Check sheet for the modelled part. Datum: model origin and axes. Units: mm. A direction names the side the tool comes from. Coordinates: 2 decimals unless noted, no trailing zeros. Order: outer loops, then holes, each group sorted by start corner. A loop starts at its lowest first (then second) coordinate and runs counter-clockwise, first axis right, second up.
1. Thickness scan on line 1 (X direction, y = 40, z = -17); line 2 (X direction, y = 68, z = 24); line 3 (Z direction, x = 15, y = 27). Record the ranges inside material, lowest first.
2. Cross-section at C-C (y = 46). Enter the section's corners in (x, z), then the cut area to 3 significant figures.
3. Cross-section at B-B (x = -26). Enter the section's corners in (y, z), then the cut area to 3 significant figures.
4. Cross-section at D-D (z = -24.5). Enter the section's corners in (x, y).
5. Set-up check for faces 5 (the flat face through (-24.669, 32, -5)), 6 (the flat face through (10, 8, 31.058)), 7 (the flat face through (-10, 23, -9.468)): record each of +Z, -Z, +X, -X, +Y, -Y from which the full face is reachable in a straight line by a thin tool's end or side.
6. Gauge pin test, flat ends, axial feed: pin 1 Ø8 at (y, z) = (22.5, -18) entering from -X; pin 2 Ø2 at (x, z) = (-22, 27) entering from +Y; pin 3 Ø2.5 at (x, z) = (-22.67, -36.97) entering from +Y. Record the tip position at first contact, or that the pin passes through.
7. Draft check along Y on faces 1 (the flat face through (44.331, 6, 26)), 2 (the cylindrical face through (-28.725, 52.482, -3.451)), 3 (the flat face through (39, 63, -5)), 4 (the flat face through (10, 63, -45)). Enter one of: released by +Y, released by -Y, zero draft, split by the parting line, or undercut.
8. Cross-section at A-A (x = 12). Enter the section's corners in (y, z).
Autodesk Inventor part; units mm, degrees
ref_plane "YZ Plane" through (0, 0, 0) normal (1, 0, 0) x (0, 1, 0)
ref_plane "XZ Plane" through (0, 0, 0) normal (0, 1, 0) x (-1, 0, 0)
ref_plane "XY Plane" through (0, 0, 0) normal (0, 0, 1) x (1, 0, 0)
sketch "Sketch1" plane through (0, 0, 0) normal (0, 1, 0) x (-1, 0, 0)
  line L0 (32.6686, 38.0315) -> (-52.3314, 38.0315)
  line L1 (-52.3314, 38.0315) -> (-52.3314, -46.9685)
  line L2 (-52.3314, -46.9685) -> (32.6686, -46.9685)
  line L3 (32.6686, -46.9685) -> (32.6686, 38.0315)
  point P0 (0, 0)
  dimension "d0" = 85
  dimension "d1" = 85
extrude "Extrusion1" add sketch "Sketch1" along normal blind 73
sketch "Sketch2" plane through (52.3314, 0, 38.0315) normal (1, 0, 0) x (0, 0, -1)
  point P0 (38.0315, 0)
sketch "Sketch3" plane through (52.3314, 0, 38.0315) normal (1, 0, 0) x (0, 0, -1)
  circle A0 centre (42.5, 23) radius 29.5
  line L0 (0, 73) -> (85, 73)
  line L1 (85, 0) -> (85, 73)
  point P0 (38.0315, 0)
  dimension "d4" = 59
  dimension "d5" = 50
  dimension "d6" = 42.5
extrude "Extrusion2" cut sketch "Sketch3" against normal blind 8
sketch "Sketch4" plane through (-32.6686, 0, -46.9685) normal (-1, 0, 0) x (0, 0, 1)
  arc A0 (60.973, 0) -> (24.027, 0) centre (42.5, 23) ccw
  circle A1 centre (42.5, 23) radius 29.5
  point P0 (46.9685, 0)
  point P1 (24.027, 0)
extrude "Extrusion3" cut sketch "Sketch4" against normal blind 8
sketch "Sketch5" plane through (0, 0, 0) normal (0, -1, 0) x (1, 0, 0)
  line L0 (-24.6686, 14.0044) -> (-24.6686, -22.9415)
  line L1 (-24.6686, -9.4685) -> (5.3314, -9.4685)
  line L2 (5.3314, -9.4685) -> (5.3314, 0.5315)
  line L3 (-4.6686, 0.5315) -> (-24.6686, 0.5315)
  line L4 (-24.6686, 0.5315) -> (-24.6686, -9.4685)
  line L5 (-4.6686, 0.5315) -> (-4.6686, 25.5315)
  line L6 (-4.6686, 25.5315) -> (5.3314, 25.5315)
  line L7 (5.3314, 25.5315) -> (5.3314, 0.5315)
  line L8 (-24.6686, -9.4685) -> (-24.6686, 0.5315)
  line L9 (44.3314, -9.4685) -> (14.3314, -9.4685)
  line L10 (14.3314, -9.4685) -> (14.3314, 0.5315)
  line L11 (24.1898, 0.5315) -> (44.3314, 0.5315)
  line L12 (24.1898, 0.5315) -> (24.3314, 25.5315)
  line L13 (24.3314, 25.5315) -> (14.3314, 25.5315)
  line L14 (14.3314, 25.5315) -> (14.3314, 0.5315)
  line L15 (44.3314, -9.4685) -> (44.3314, 0.5315)
  line L16 (44.3314, -22.9415) -> (44.3314, 14.0044)
  point P0 (0, 0)
  dimension "d13" = 13.473
  dimension "d35" = 10
  dimension "d36" = 9
  dimension "d37" = 10
sketch "Sketch6" plane through (-24.6686, 0, -46.9685) normal (-1, 0, 0) x (0, 0, 1)
  arc A0 (60.973, 0) -> (24.027, 0) centre (42.5, 23) ccw
  line L0 (42.5, 23) -> (131.4973, 23)
  point P0 (46.9685, 0)
extrude "Extrusion4" cut sketch "Sketch5" against normal blind 29
sketch "Sketch7" plane through (0, 0, 0) normal (0, -1, 0) x (1, 0, 0)
  line L0 (-24.6686, -22.9415) -> (44.3314, -22.9415)
  line L1 (44.3314, -22.9415) -> (44.3314, 31.0585)
  line L2 (44.3314, 31.0585) -> (-24.6686, 31.0585)
  line L3 (-24.6686, 31.0585) -> (-24.6686, -22.9415)
  point P0 (0, 0)
  dimension "d19" = 69
  dimension "d20" = 54
extrude "Extrusion5" cut sketch "Sketch7" against normal blind 17
sketch "Sketch8" plane through (0, 17, 0) normal (0, -1, 0) x (1, 0, 0)
  circle A0 centre (-15.6686, -13.9415) radius 2
  circle A1 centre (-15.6686, 11.0585) radius 2
  circle A2 centre (34.3314, 11.0585) radius 2
  circle A3 centre (34.3314, -13.9415) radius 2
  line L0 (-26.1879, -23.917) -> (41.8121, -23.917)
  line L1 (-24.6686, 31.0585) -> (44.3314, 31.0585)
  line L2 (-24.6686, 31.0585) -> (44.3314, 31.0585)
  line L3 (44.3314, 31.0585) -> (44.3314, -22.9415)
  line L4 (44.3314, -22.9415) -> (-24.6686, -22.9415)
  line L5 (-24.6686, -22.9415) -> (-24.6686, 31.0585)
  point P0 (0, 0)
  point P1 (-18.7833, -12.5016)
  dimension "d23" = 4
  dimension "d24" = 4
  dimension "d25" = 4
  dimension "d26" = 4
  dimension "d27" = 50
  dimension "d28" = 25
  dimension "d31" = 9
  dimension "d32" = 9
extrude "Extrusion6" cut sketch "Sketch8" against normal blind 5.8 contours A0 | A1 | A2 | A3
sketch "Sketch9" plane through (0, 29, 0) normal (0, -1, 0) x (1, 0, 0)
  line L0 (24.1898, 0.5315) -> (24.3314, 25.5315)
  line L1 (14.3314, 25.5315) -> (14.3314, -9.4685)
  line L2 (24.3314, 25.5315) -> (14.3314, 25.5315)
  line L3 (14.3314, 25.5315) -> (14.3314, 19.5315)
  line L4 (14.3314, 19.5315) -> (24.3314, 19.5315)
  line L5 (24.3314, 19.5315) -> (24.3314, 25.5315)
  line L6 (5.3314, -9.4685) -> (5.3314, 25.5315)
  line L7 (5.3314, 25.5315) -> (-14.6686, 25.5315)
  line L8 (-14.6686, 25.5315) -> (-14.6686, 19.5315)
  line L9 (-14.6686, 19.5315) -> (5.3314, 19.5315)
  line L10 (5.3314, 19.5315) -> (5.3314, 25.5315)
  point P0 (0, 0)
  point P1 (24.2974, 19.5315)
  dimension "d39" = 20
  dimension "d40" = 6
  dimension "d47" = 10
extrude "Extrusion7" cut sketch "Sketch9" against normal blind 61.25 contours L4 L1 L2 L0 | L9 L8 L7 L6
sketch "Sketch10" plane through (0, 73, 0) normal (0, 1, 0) x (1, 0, 0)
  line L0 (52.3314, 46.9685) -> (-32.6686, 46.9685)
  line L1 (-10.1686, 46.9685) -> (29.8314, 46.9685)
  line L2 (29.8314, 46.9685) -> (29.8314, -35.0315)
  line L3 (29.8314, -35.0315) -> (-10.1686, -35.0315)
  line L4 (-10.1686, -35.0315) -> (-10.1686, 46.9685)
  line L5 (-32.6686, 46.9685) -> (-32.6686, -38.0315)
  point P0 (0, 0)
  dimension "d43" = 40
  dimension "d44" = 82
  dimension "d51" = 22.5
sketch "Sketch11" plane through (0, 29, 0) normal (0, -1, 0) x (1, 0, 0)
  line L0 (24.2974, 19.5315) -> (14.3314, 19.5315)
  line L1 (14.3314, 19.5315) -> (34.3314, 19.5315)
  line L2 (34.3314, 19.5315) -> (34.3314, 25.5315)
  line L3 (34.3314, 25.5315) -> (14.3314, 25.5315)
  line L4 (14.3314, 25.5315) -> (14.3314, 19.5315)
  point P0 (0, 0)
  dimension "d48" = 20
extrude "Extrusion8" cut sketch "Sketch11" against normal blind 61.25
extrude "Extrusion9" cut sketch "Sketch10" against normal blind 40
sketch "Sketch12" plane through (0, 73, 0) normal (0, 1, 0) x (1, 0, 0)
  line L0 (-56.5689, -78.065) -> (64.3856, -78.065)
  line L1 (64.3856, -78.065) -> (64.3856, 116.3261)
  line L2 (64.3856, 116.3261) -> (-56.5689, 116.3261)
  line L3 (-56.5689, 116.3261) -> (-56.5689, -78.065)
  point P0 (0, 0)
extrude "Extrusion10" cut sketch "Sketch12" against normal blind 10
sketch "Sketch14" plane through (0, 63, 0) normal (0, 1, 0) x (1, 0, 0)
  circle A0 centre (42.3314, -28.0315) radius 2
  circle A1 centre (-22.6686, -28.0315) radius 2
  circle A2 centre (-22.6686, 36.9685) radius 2
  circle A3 centre (42.3314, 36.9685) radius 2
  line L0 (52.3314, 46.9685) -> (52.3314, -38.0315)
  line L1 (52.3314, -38.0315) -> (-32.6686, -38.0315)
  line L2 (-32.6686, -38.0315) -> (-32.6686, 46.9685)
  point P0 (0, 0)
  dimension "d56" = 4
  dimension "d57" = 4
  dimension "d58" = 4
  dimension "d59" = 4
  dimension "d60" = 65
  dimension "d61" = 65
  dimension "d62" = 10
  dimension "d63" = 10
  dimension "d64" = 10
extrude "Extrusion11" cut sketch "Sketch14" against normal blind 5.8
sketch "Sketch15" plane through (0, 63, 0) normal (0, 1, 0) x (1, 0, 0)
  line L0 (-32.6686, 46.9685) -> (-32.6686, 22.9415)
  line L1 (-32.6686, 46.9685) -> (-29.6686, 46.9685)
  line L2 (52.3314, 46.9685) -> (-32.6686, 46.9685)
  line L3 (-29.6686, 43.9685) -> (-29.6686, -35.0315)
  line L4 (-32.6686, -38.0315) -> (-32.6686, 46.9685)
  line L5 (-32.6686, -38.0315) -> (-29.6686, -38.0315)
  line L6 (-29.6686, 46.9685) -> (-32.6686, 46.9685)
  line L7 (-32.6686, 46.9685) -> (-32.6686, -38.0315)
  line L8 (52.3314, 46.9685) -> (52.3314, -38.0315)
  line L9 (52.3314, -38.0315) -> (-29.6686, -38.0315)
  line L10 (-29.6686, -35.0315) -> (49.3314, -35.0315)
  line L11 (52.3314, -35.0315) -> (52.3314, -38.0315)
  line L12 (52.3314, 46.9685) -> (49.3314, 46.9685)
  line L13 (49.3314, 43.9685) -> (49.3314, -35.0315)
  line L14 (49.3314, -38.0315) -> (52.3314, -38.0315)
  line L15 (52.3314, -38.0315) -> (52.3314, 46.9685)
  line L16 (49.3314, 46.9685) -> (-29.6686, 46.9685)
  line L17 (-29.6686, 43.9685) -> (49.3314, 43.9685)
  point P0 (0, 0)
  dimension "d67" = 3
  dimension "d69" = 3
  dimension "d70" = 3
extrude "Extrusion12" add sketch "Sketch15" along normal blind 20
sketch "Sketch16" plane through (0, 29, 0) normal (0, 1, 0) x (1, 0, 0)
  line L0 (-14.6686, -25.5315) -> (-14.6686, -19.5315)
  line L1 (5.3314, 9.4685) -> (5.3314, -25.5315)
  line L2 (-14.6686, -19.5315) -> (5.3314, -19.5315)
  line L3 (5.3314, -19.5315) -> (5.3314, -25.5315)
  line L4 (5.3314, -25.5315) -> (-14.6686, -25.5315)
  line L5 (-14.6686, -25.5315) -> (-14.6686, -19.5315)
  line L6 (24.2974, -19.5315) -> (14.3314, -19.5315)
  line L7 (34.3314, -25.5315) -> (24.3314, -25.5315)
  line L8 (14.3314, -19.5315) -> (34.3314, -19.5315)
  line L9 (34.3314, -19.5315) -> (34.3314, -25.5315)
  line L10 (34.3314, -25.5315) -> (14.3314, -25.5315)
  line L11 (14.3314, -25.5315) -> (14.3314, -19.5315)
  point P0 (0, 0)
  point P1 (5.3314, -19.5315)
extrude "Extrusion13" cut sketch "Sketch16" against normal through all
sketch "Sketch17" plane through (0, 0, 0) normal (0, -1, 0) x (1, 0, 0)
  point P0 (0, 0)
sketch "Sketch18" plane through (0, 17, 0) normal (0, -1, 0) x (1, 0, 0)
  line L0 (5.3314, 19.5315) -> (5.3314, -9.4685)
  line L1 (5.3314, -9.4685) -> (16.5671, -9.4685)
  line L2 (16.5671, -9.4685) -> (16.5671, 0.5747)
  line L3 (16.5671, 0.5747) -> (5.3314, 0.5747)
  line L4 (5.3314, 0.5747) -> (5.3314, -9.4685)
  point P0 (0, 0)
properties part number "RobotBase"
Data:
1. line 1: x = -24.67 to -10.17, 29.83 to 44.33
1. line 2: x = -32.67 to -29.67, 49.33 to 52.33
1. line 3: z = -46.97 to -9.47, 25.53 to 38.03
2. outline: (-32.67, -46.97) - (-10.17, -46.97) - (-10.17, 19.53) - (-14.67, 19.53) - (-14.67, 25.53) - (-10.17, 25.53) - (-10.17, 35.03) - (29.83, 35.03) - (29.83, 25.53) - (34.33, 25.53) - (34.33, 19.53) - (29.83, 19.53) - (29.83, -46.97) - (52.33, -46.97) - (52.33, -22.94) - (44.33, -22.94) - (44.33, 14) - (52.33, 14) - (52.33, 38.03) - (-32.67, 38.03) - (-32.67, 14) - (-24.67, 14) - (-24.67, -22.94) - (-32.67, -22.94) - close
2. area: 3,300 mm2
3. outline: (0, -46.97) - (83, -46.97) - (83, -43.97) - (63, -43.97) - (63, 35.03) - (83, 35.03) - (83, 38.03) - (0, 38.03) - (0, 14) arc R29.5 cw (long way) to (0, -22.94) - close
3. area: 2,910 mm2
4. outline: (-32.67, 0) - (52.33, 0) - (52.33, 1.34) - (44.33, 1.34) - (44.33, 44.66) - (52.33, 44.66) - (52.33, 83) - (49.33, 83) - (49.33, 63) - (29.83, 63) - (29.83, 33) - (-10.17, 33) - (-10.17, 63) - (-29.67, 63) - (-29.67, 83) - (-32.67, 83) - (-32.67, 44.66) - (-24.67, 44.66) - (-24.67, 1.34) - (-32.67, 1.34) - close
5. face 5: -X
5. face 6: -Y
5. face 7: -X, -Y
6. pin 1: stops at x = -24.67
6. pin 2: stops at y = 63
6. pin 3: stops at y = 57.2
7. face 1: zero draft
7. face 2: undercut
7. face 3: released by +Y
7. face 4: undercut
8. outline: (0, -46.97) - (33, -46.97) - (33, 35.03) - (83, 35.03) - (83, 38.03) - (0, 38.03) - (0, 31.06) - (17, 31.06) - (17, -22.94) - (0, -22.94) - close; (63, -46.97) - (83, -46.97) - (83, -43.97) - (63, -43.97) - close
